For this review, use the dimensioned drawing (mm, ordinates from the lowest corner) and the shaded views. A direction names the side the tool comes from. Coordinates: 2 decimals unless noted, no trailing zeros. Order: outer loops, then holes, each group sorted by start corner. A loop starts at its lowest first (then second) coordinate and runs counter-clockwise, first axis right, second up. Notation, with made-up numbers: (-21.75, -28.5) -> (36.25, -28.5) arc R18 ccw to (36.25, -16.5) -> close; hole circle Ø8 at (68.25, -22.5). An arc over 180 degrees is marked (long way). Return JSON: item names as keys, results as strings. Group by question number.
Item 1: For line 1 along Z through (x, y) = (39.17, 0.4); line 2 along X through (y, z) = (9.5, 100.5); line 3 along X through (y, z) = (11, 21), list the stretches that pass through material, from the lowest coordinate up.
Item 2: Take a section at D-D (z = 17). Write out the cut boundary in (x, y).
Item 3: Take a section at B-B (z = 93.8). Write out the cut boundary in (x, y).
Item 4: Machinability: for the marked faces 1 and 2, which of the approach directions +Z, -Z, +X, -X, +Y, -Y give a long, thin tool a straight path to every point of the face, cutting with its end or side? Answer none if there is none.
Item 5: Insertion check: pin 1 (12 mm diameter, centred on x = 27, z = 23.5, fed in from +Y); pin 2 (1.5 mm diameter, centred on x = 1.5, y = 15, fed in from -Z). Each pin has a flat end and moves straight along its axis. Give the tip position at first contact, or say it passes through.
Item 6: Take a section at A-A (y = 9.5). Write out the cut boundary in (x, z), then the cut area to 3 significant figures.
Item 7: Draft analysis for pull direction X (two halves, no side actions). For the marked faces 3, 4 and 5, state which applies: +X half, -X half, draft (parallel to the pull), parting line (faces both ways), or undercut.
Item 8: Take a section at C-C (x = 18.5). Write out the cut boundary in (y, z), then the cut area to 3 significant figures.
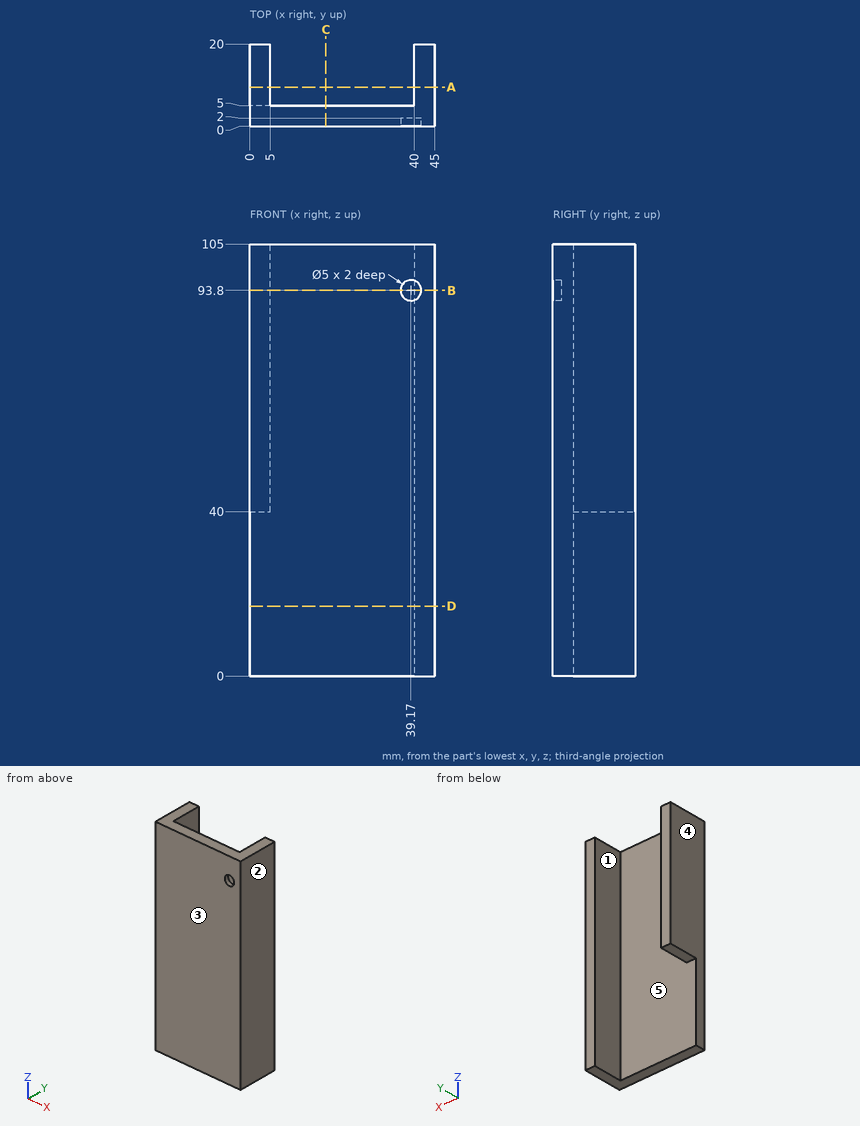
Findings below:
{
 "1": {"line 1": "z = 0 to 91.3, 96.3 to 105", "line 2": "x = 0 to 5, 40 to 45", "line 3": "x = 40 to 45"},
 "2": {"outline": "(0, 0) -> (45, 0) -> (45, 20) -> (40, 20) -> (40, 5) -> (0, 5) -> close"},
 "3": {"outline": "(0, 0) -> (36.67, 0) -> (36.67, 2) -> (41.67, 2) -> (41.67, 0) -> (45, 0) -> (45, 20) -> (40, 20) -> (40, 5) -> (5, 5) -> (5, 20) -> (0, 20) -> close"},
 "4": {"face 1": "+Z, -Z, +Y", "face 2": "+Z, -Z, +X, +Y, -Y"},
 "5": {"pin 1": "stops at y = 5", "pin 2": "stops at z = 40"},
 "6": {"outline": "(0, 40) -> (5, 40) -> (5, 105) -> (0, 105) -> close; (40, 0) -> (45, 0) -> (45, 105) -> (40, 105) -> close", "area": "850 mm2"},
 "7": {"face 3": "draft", "face 4": "-X half", "face 5": "undercut"},
 "8": {"outline": "(0, 0) -> (5, 0) -> (5, 105) -> (0, 105) -> close", "area": "525 mm2"}
}
